Can you work these out from the model? Positions are in its coordinate system, mm. A direction names the side the tool comes from. Give positions to 0.01 mm unless a question says otherwise; leave off trailing zeros. Order: outer loops, then holes, each group sorted by start corner. A loop starts at its lowest first (then second) coordinate and runs counter-clockwise, first axis right, second up. Notation, with made-up numbers: (-16, 54.5) - (23, 54.5) arc R27 cw to (23, 78.5) - close; hole circle Ø8 at (31, 42.5). An arc over 180 degrees is marked (long way). Return JSON: item names as keys, results as strings.
```python
from build123d import *

# Parameters (mm, degrees)
SKETCH1_R               = 49.4411
BOSS_EXTRUDE2_DEPTH     = 9.525
SKETCH4_R               = 50.546
SKETCH4_R_2             = 47.625
CUT_EXTRUDE2_DEPTH      = 4.7625
CUT_EXTRUDE4_DEPTH      = 71.566070908
CUT_EXTRUDE4_DEPTH_BACK = 71.566070908
SKETCH5_R               = 4.826
CUT_EXTRUDE5_DEPTH      = 71.566070908
CUT_EXTRUDE5_DEPTH_BACK = 71.566070908
SKETCH6_W               = 12.827
SKETCH6_H               = 6.477


with BuildPart() as part:
    # Sketch1 → Boss-Extrude2 (new body)
    with BuildSketch(Plane(origin=(0, 0, 0), x_dir=(1, 0, 0), z_dir=(0, 1, 0))):
        with Locations(Location((0, 0, 0), (0, 0, 90))):
            Circle(SKETCH1_R)
    extrude(amount=BOSS_EXTRUDE2_DEPTH)

    # Sketch4 → Cut-Extrude2 (cut)
    with BuildSketch(Plane(origin=(0, 9.525, 0), x_dir=(1, 0, 0), z_dir=(0, 1, 0))):
        Circle(SKETCH4_R)
        with Locations(Location((0, 0, 0), (0, 0, 270))):
            Circle(SKETCH4_R_2, mode=Mode.SUBTRACT)
    extrude(amount=-CUT_EXTRUDE2_DEPTH, mode=Mode.SUBTRACT)

    # Sketch5 → Cut-Extrude4 (cut, two sides: drawn at the far end of the back side and taken through both)
    with BuildSketch(Plane.XZ.offset(-CUT_EXTRUDE4_DEPTH_BACK)):
        with Locations(Location((-0.0635, 30.162076648, 0), (0, 0, 270))):
            Circle(SKETCH5_R)
        with Locations(Location((-0.0635, -30.162076648, 0), (0, 0, 270))):
            Circle(SKETCH5_R)
        with Locations(Location((-38.1, 0, 0), (0, 0, 270))):
            Circle(SKETCH5_R)
        with Locations(Location((38.1, 0, 0), (0, 0, 270))):
            Circle(SKETCH5_R)
    extrude(amount=CUT_EXTRUDE4_DEPTH + CUT_EXTRUDE4_DEPTH_BACK, mode=Mode.SUBTRACT)

    # Sketch6 → Cut-Extrude5 (cut, two sides: drawn at the far end of the back side and taken through both)
    with BuildSketch(Plane(origin=(0, 9.525, 0), x_dir=(1, 0, 0), z_dir=(0, 1, 0)).offset(-CUT_EXTRUDE5_DEPTH_BACK)):
        with Locations((25.3365, 15.9385)):
            Rectangle(SKETCH6_W, SKETCH6_H)
    extrude(amount=CUT_EXTRUDE5_DEPTH + CUT_EXTRUDE5_DEPTH_BACK, mode=Mode.SUBTRACT)


solid = part.part
```
1. On a 3-axis mill with a long thin cutter (end or side, diameter ignored), from which of +Z, -Z, +X, -X, +Y, -Y can I reach the whole of each face in a straight line? I mean faces 1 (the face through (-26, 4.762, -41)), 2 (the face through (-1, 9.525, 1)), 3 (the face through (25, 5, -12.7)). Say none if no direction works.
Checks:
{"face 1": "+Y", "face 2": "+Z, -Z, +X, -X, +Y", "face 3": "+Y, -Y"}
2. Suppose I cut it at B-B (x = -36). List the corners of the cut face in (y, z) for me (1 decimal).
Checks:
{"outline": "(0, -33.9) - (4.8, -33.9) - (4.8, -31.2) - (9.5, -31.2) - (9.5, -4.3) - (0, -4.3) - close; (0, 4.3) - (9.5, 4.3) - (9.5, 31.2) - (4.8, 31.2) - (4.8, 33.9) - (0, 33.9) - close"}
3. If I drill on L1, parallel to X at y = 3.5, z = 0; L2, parallel to X at y = 5.5, z = 0 (3 decimals); L3, parallel to Y at x = 25.5, z = -41.5, over which ranges is the centre line in solid material (lowest first)? Write a range as [from, to].
Checks:
{"L1": "[-49.44, -42.93], [-33.27, 33.27], [42.93, 49.44]", "L2": "[-47.625, -42.926], [-33.274, 33.274], [42.926, 47.625]", "L3": "[0, 4.76]"}
4. Suppose I cut it at A-A (z = 0). List the corners of the cut face in (x, y) for me (1 decimal).
Checks:
{"outline": "(-49.4, 0) - (-42.9, 0) - (-42.9, 9.5) - (-47.6, 9.5) - (-47.6, 4.8) - (-49.4, 4.8) - close; (-33.3, 0) - (33.3, 0) - (33.3, 9.5) - (-33.3, 9.5) - close; (42.9, 0) - (49.4, 0) - (49.4, 4.8) - (47.6, 4.8) - (47.6, 9.5) - (42.9, 9.5) - close"}
5. Suppose I cut it at D-D (x = 2.5). List the corners of the cut face in (y, z) for me (1 decimal), plus the area to 3 significant figures.
Checks:
{"outline": "(0, -49.4) - (4.8, -49.4) - (4.8, -47.6) - (9.5, -47.6) - (9.5, -34.3) - (0, -34.3) - close; (0, -26.1) - (9.5, -26.1) - (9.5, 26.1) - (0, 26.1) - close; (0, 34.3) - (9.5, 34.3) - (9.5, 47.6) - (4.8, 47.6) - (4.8, 49.4) - (0, 49.4) - close", "area": "768 mm^2"}
6. Suppose I cut it at C-C (y = 7.5). State how many separate pieces and enclosed holes the cut face has, plus the area to 3 significant figures.
Checks:
{"separate pieces": "1", "enclosed holes": "5", "area": "6,750 mm^2"}
7. Thinking about a two-plate mould opening in Z: for faces 4 (the face through (-1, 0, 1)), 5 (the face through (-46.492, 7.177, -10.324)), 6 (the face through (42.885, 4.829, 0.628)), which applies, +Z half, -Z half, draft (parallel to the pull), parting line (faces both ways), or undercut?
Checks:
{"face 4": "draft", "face 5": "parting line", "face 6": "undercut"}
8. For pin 1 Ø1 at (x, z) = (-32.5, 0) entering from -Y; pin 2 Ø5 at (y, z) = (4, -16) entering from -X; pin 3 Ø3 at (y, z) = (5, -21) entering from -X; pin 4 Ø1.9 at (y, z) = (5, -17) entering from +X, each with a flat end and sliding along its axis, tell me the tip position at first contact or that it passes through.
Checks:
{"pin 1": "y = 0", "pin 2": "x = -47.56", "pin 3": "x = -45.43", "pin 4": "x = 46.75"}
